Read the model definition and answer for the solid it produces. Units are mm, in the model's axes. A direction names the side the tool comes from. Coordinates: 2 decimals unless noted, no trailing zeros. Write each loop counter-clockwise with the first axis right and the second up, starting at its lowest first coordinate (ties: lowest second). Pieces come first, ordered by that corner, then holes. Notation, with made-up numbers: (69, -24) - (100, -24) arc R38 cw to (100, 15) - close; hole circle Ø11 at (-37, -18.75). An arc over 180 degrees is marked (long way). Return JSON: item names as keys, results as strings.
Autodesk Inventor part; units mm, degrees
ref_plane "YZ Plane" through (0, 0, 0) normal (1, 0, 0) x (0, 1, 0)
ref_plane "XZ Plane" through (0, 0, 0) normal (0, 1, 0) x (-1, 0, 0)
ref_plane "XY Plane" through (0, 0, 0) normal (0, 0, 1) x (1, 0, 0)
sketch "Sketch1" plane through (0, 0, 0) normal (0, 0, 1) x (1, 0, 0)
  line L0 (0, 0) -> (0, 90)
  line L1 (0, 90) -> (19.2, 90)
  line L2 (19.2, 90) -> (19.2, 37.65)
  line L3 (19.2, 37.65) -> (35.07, 37.65)
  line L4 (35.07, 37.65) -> (35.07, 90)
  line L5 (35.07, 90) -> (54.27, 90)
  line L6 (54.27, 90) -> (54.27, 0)
  line L7 (54.27, 0) -> (35.07, 0)
  line L8 (35.07, 0) -> (35.07, 26.67)
  line L9 (35.07, 26.67) -> (19.2, 26.67)
  line L10 (19.2, 26.67) -> (19.2, 0)
  line L11 (0, 0) -> (19.2, 0)
  dimension "d0" = 90
  dimension "d1" = 19.2
  dimension "d2" = 52.35
  dimension "d3" = 15.87
  dimension "d4" = 19.2
  dimension "d5" = 26.67
extrude "Extrusion1" add sketch "Sketch1" along normal blind 20.67
sketch "Sketch2" plane through (19.2, 37.65, 0) normal (0, 1, 0) x (1, 0, 0)
  line L0 (15.87, 0) -> (0, 0)
  line L1 (11.39, 0) -> (4.49, 0)
  line L2 (4.49, 0) -> (4.49, -4.29)
  line L3 (4.49, -4.29) -> (11.39, -4.29)
  line L4 (11.39, -4.29) -> (11.39, 0)
  point P0 (-19.2, 0)
  dimension "d8" = 6.9
  dimension "d9" = 4.29
extrude "Extrusion2" add sketch "Sketch2" along normal blind 27.15
sketch "Sketch3" plane through (23.69, 37.65, 4.29) normal (0, 0, 1) x (1, 0, 0)
  line L0 (6.9, 0) -> (0, 0)
  line L1 (0, 27.15) -> (6.9, 27.15)
  line L2 (0, 0) -> (0, 27.15)
  line L3 (6.9, 27.15) -> (9.7769, 2.4369)
  line L4 (6.9, 27.15) -> (31.78, 27.15) construction
  line L5 (9.7769, 2.4369) -> (6.9, 2.4369)
  line L6 (6.9, 0) -> (6.9, 27.15)
  line L7 (0, 2.4369) -> (-2.877, 2.4369)
  line L8 (-2.877, 2.4369) -> (0, 27.15)
  point P0 (-23.69, -37.65)
  dimension "d12" = 24.88
  dimension "d13" = 83.36
  dimension "d14" = 2.877
extrude "Extrusion3" add sketch "Sketch3" against normal blind 4.29
sketch "Sketch4" plane through (19.2, 26.67, 0) normal (0, -1, 0) x (1, 0, 0)
  line L0 (0, 0) -> (0, 20.67)
  line L1 (0, 0) -> (4.49, 0)
  line L2 (4.48, 0) -> (11.38, 0)
  line L3 (11.38, 0) -> (11.38, 4.29)
  line L4 (11.38, 4.29) -> (4.48, 4.29)
  line L5 (4.48, 4.29) -> (4.48, 0)
  point P0 (-19.2, 0)
  dimension "d17" = 6.9
  dimension "d18" = 4.29
  dimension "d19" = 4.48
extrude "Extrusion4" add sketch "Sketch4" along normal blind 18.76
sketch "Sketch5" plane through (23.68, 26.67, 4.29) normal (0, 0, 1) x (1, 0, 0)
  line L0 (0, 0) -> (6.9, 0)
  line L1 (0, 0) -> (0, -18.76)
  line L2 (6.9, -18.76) -> (0, -18.76)
  line L3 (0, -18.76) -> (-2.87, -2.3288)
  line L4 (-4.48, -26.67) -> (-4.48, 0)
  line L5 (-2.87, -2.3288) -> (0, -2.3288)
  line L6 (6.9, 0) -> (6.9, -18.76)
  line L7 (6.9, -2.3288) -> (9.777, -2.3288)
  line L8 (9.777, -2.3288) -> (6.9, -18.76)
  point P0 (-23.68, -26.67)
  dimension "d22" = 16.68
  dimension "d23" = 1.61
  dimension "d24" = 2.877
extrude "Extrusion5" add sketch "Sketch5" against normal blind 4.29
sketch "Sketch6" plane through (0, 0, 20.67) normal (0, 0, 1) x (1, 0, 0)
  line L0 (0.93, 0.93) -> (0.93, 89.07)
  line L1 (0, 90) -> (19.2, 90)
  line L2 (0.93, 89.07) -> (18.27, 89.07)
  line L3 (18.27, 89.07) -> (18.27, 36.72)
  line L4 (18.27, 36.72) -> (36, 36.72)
  line L5 (36, 36.72) -> (36, 89.07)
  line L6 (36, 89.07) -> (53.34, 89.07)
  line L7 (53.34, 89.07) -> (53.34, 0.93)
  line L8 (53.34, 0.93) -> (36, 0.93)
  line L9 (36, 0.93) -> (36, 27.6)
  line L10 (36, 27.6) -> (18.27, 27.6)
  line L11 (18.27, 27.6) -> (18.27, 0.93)
  line L12 (18.27, 0.93) -> (0.93, 0.93)
  dimension "d27" = 88.14
  dimension "d28" = 17.34
  dimension "d29" = 52.35
  dimension "d30" = 17.73
  dimension "d31" = 52.35
  dimension "d32" = 17.34
  dimension "d33" = 88.14
  dimension "d34" = 26.67
extrude "Extrusion6" cut sketch "Sketch6" against normal blind 0.62
properties part number "print Helix V1"
(1) A flat-ended cylindrical pin translates along its axis: P1, Ø3, axis at x = 48.5, y = 10, coming from the +Z side. Find the tip coordinate at first contact, or state that the pin passes through.
Answer:
{"P1": "z = 20.05"}
(2) A cutting plane is placed at C-C (y = 78.5). Determine the outline of the cut face in (x, z), and give its area (3 significant figures).
Answer:
{"outline": "(0, 0) - (19.2, 0) - (19.2, 20.67) - (18.27, 20.67) - (18.27, 20.05) - (0.93, 20.05) - (0.93, 20.67) - (0, 20.67) - close; (35.07, 0) - (54.27, 0) - (54.27, 20.67) - (53.34, 20.67) - (53.34, 20.05) - (36, 20.05) - (36, 20.67) - (35.07, 20.67) - close", "area": "772 mm²"}
(3) A cutting plane is placed at D-D (z = 2.25). Determine the outline of the cut face in (x, y).
Answer:
{"outline": "(0, 0) - (19.2, 0) - (19.2, 26.67) - (23.68, 26.67) - (23.68, 24.34) - (20.81, 24.34) - (23.68, 7.91) - (30.58, 7.91) - (33.46, 24.34) - (30.58, 24.34) - (30.58, 26.67) - (35.07, 26.67) - (35.07, 0) - (54.27, 0) - (54.27, 90) - (35.07, 90) - (35.07, 37.65) - (30.59, 37.65) - (30.59, 40.09) - (33.47, 40.09) - (30.59, 64.8) - (23.69, 64.8) - (20.81, 40.09) - (23.69, 40.09) - (23.69, 37.65) - (19.2, 37.65) - (19.2, 90) - (0, 90) - close"}
(4) A cutting plane is placed at A-A (y = 13). Determine the outline of the cut face in (x, z), and give its area (3 significant figures).
Answer:
{"outline": "(0, 0) - (19.2, 0) - (19.2, 20.67) - (18.27, 20.67) - (18.27, 20.05) - (0.93, 20.05) - (0.93, 20.67) - (0, 20.67) - close; (22.79, 0) - (31.47, 0) - (31.47, 4.29) - (22.79, 4.29) - close; (35.07, 0) - (54.27, 0) - (54.27, 20.67) - (53.34, 20.67) - (53.34, 20.05) - (36, 20.05) - (36, 20.67) - (35.07, 20.67) - close", "area": "809 mm²"}
(5) Which of the six approach directions +Z, -Z, +X, -X, +Y, -Y give full straight-line access (tool end or side, diameter ignored) to faces 4 (the face through (27, 51, 4.29)), 5 (the face through (32, 24.341, 2)), 6 (the face through (19.2, 64, 10)), 7 (the face through (45, 90, 10)), 8 (the face through (22.265, 16.011, 2.175))?
Answer:
{"face 4": "+Z, +Y", "face 5": "+Z, -Z", "face 6": "+Z, -Z, +Y", "face 7": "+Z, -Z, +X, -X, +Y", "face 8": "+Z, -Z, -Y"}
(6) Determine the mould class of faces 1 (the face through (30.58, 26, 2)), 2 (the face through (27, 46, 0)), 3 (the face through (0, 44, 10)) for opening direction X: +X half, -X half, draft (parallel to the pull), parting line (faces both ways), or undercut.
Answer:
{"face 1": "undercut", "face 2": "draft", "face 3": "-X half"}
(7) A cutting plane is placed at B-B (x = 17). Determine the outline of the cut face in (y, z).
Answer:
{"outline": "(0, 0) - (90, 0) - (90, 20.67) - (89.07, 20.67) - (89.07, 20.05) - (0.93, 20.05) - (0.93, 20.67) - (0, 20.67) - close"}
(8) Straight lines are drawn through the part: line 1 (X direction, y = 40.5, z = 16.5); line 2 (X direction, y = 63.5, z = 3); line 3 (Z direction, x = 27, y = 63). For each, find the intervals that lie inside material, in ascending order. Write a range as from..to.
Answer:
{"line 1": "0..19.2, 35.07..54.27", "line 2": "0..19.2, 23.54..30.74, 35.07..54.27", "line 3": "0..4.29"}
